Check sheet for the modelled part. Datum: model origin and axes. Units: mm. A direction names the side the tool comes from. Round coordinates to 2 decimals unless told otherwise and drop trailing zeros. Write each loop counter-clockwise with the first axis right and the second up, starting at its lowest first coordinate (ties: lowest second). Pieces come first, ordered by that corner, then holes. Notation, with made-up numbers: (-33, 70) - (0, 70) arc R16 ccw to (0, 91) - close; hole circle Ø1 at (45.25, 81.25). An arc over 180 degrees is marked (long way). Use one line per item in the form item = value. Start each with the question number.
1) Scan lines: probe 1 along Z at (x, y) = (4, -72.5); probe 2 along X at (y, z) = (1, 16.5); probe 3 along X at (y, z) = (12.5, 9). Record each from-to range of solid material in increasing order.
2) Set-up check for faces 1 (the face through (-28.98, -23.08, -22.23)), 2 (the face through (-7, -86, -5.272)), 3 (the face through (0, 28, 38.728)): record each of +Z, -Z, +X, -X, +Y, -Y from which the full face is reachable in a straight line by a thin tool's end or side.
3) Section check C-C (x = -7.5). Record the boundary of the cut face in (y, z), then the cut area to 3 significant figures.
4) Gauge pin test, flat end, axial feed: P1, Ø6, axis at x = 12.5, y = -101.5, coming from the +Z side. Record the tip position at first contact, or that the pin passes through.
5) Section check D-D (y = 49). Record the boundary of the cut face in (x, z), then the cut area to 3 significant figures.
6) Section check A-A (y = -44). Record the boundary of the cut face in (x, z), then the cut area to 3 significant figures.
7) Section check B-B (z = -31). Record the boundary of the cut face in (x, y).
8) Draft check along X on faces 4 (the face through (-35.266, -2, 17)), 5 (the face through (6.61, -51.35, 17.04)), 6 (the face through (-32, 91, -29)). Enter one of: +X half, -X half, draft (parallel to the pull), parting line (faces both ways), or undercut.
from build123d import *

# Parameters (mm, degrees)
F0_W     = 70.53198
F0_H     = 77.455252
F1_DEPTH = 134
F3_DEPTH = 44
F5_DEPTH = 225


with BuildPart() as f1:
    # F0 (on Front) → F1 (new body, symmetric)
    with BuildSketch(Plane.XZ):
        Rectangle(F0_W, F0_H)
    extrude(amount=F1_DEPTH, both=True)

    # F2 (on face) → F3 (cut)
    with BuildSketch(Plane.XY.offset(38.727626)):
        Polygon((-22.860736, 33.643957), (-22.860736, -134), (35.26599, -134), align=None)
    extrude(amount=-F3_DEPTH, mode=Mode.SUBTRACT)

    # F4 (on face) → F5 (cut)
    with BuildSketch(Plane.XZ.offset(134)):
        Polygon((-22.860736, -38.727626), (-35.26599, -5.272374), (-35.26599, -38.727626), align=None)
    extrude(amount=-F5_DEPTH, mode=Mode.SUBTRACT)


solid = f1.part
Results are:
q1.probe_1 = -38.73 to -5.27
q1.probe_2 = -35.27 to -22.86, -11.54 to 35.27
q1.probe_3 = -35.27 to -22.86, -15.53 to 35.27
q2.face_1 = -Z, -X, -Y
q2.face_2 = +Z, -Y
q2.face_3 = +Z, +X, -X, +Y, -Y
q3.outline = (-134, -38.73) - (134, -38.73) - (134, 38.73) - (-10.66, 38.73) - (-10.66, -5.27) - (-134, -5.27) - close
q3.area = 15,300 mm²
q4.P1 = -5.27
q5.outline = (-35.27, -5.27) - (-22.86, -38.73) - (35.27, -38.73) - (35.27, 38.73) - (-35.27, 38.73) - close
q5.area = 5,260 mm²
q6.outline = (-35.27, -5.27) - (-22.86, -38.73) - (35.27, -38.73) - (35.27, 38.73) - (4.06, 38.73) - (4.06, -5.27) - (-22.86, -5.27) - (-22.86, 38.73) - (-35.27, 38.73) - close
q6.area = 4,070 mm²
q7.outline = (-35.27, 91) - (-25.73, 91) - (-25.73, -134) - (35.27, -134) - (35.27, 134) - (-35.27, 134) - close
q8.face_4 = -X half
q8.face_5 = undercut
q8.face_6 = draft
